Source: CAD feature listing. Evaluate the final solid. Frame: model axes, mm. A direction names the side the tool comes from. Round coordinates to 2 decimals unless told otherwise and drop trailing zeros. Loops run counter-clockwise (first coordinate to the right, second up) from the corner with the lowest first, then second, coordinate; pieces in that order, holes last. Notation, with made-up numbers: M 76,84.5 L 134,84.5 A25 ccw 134,122.5 Z; hole C 5.5,46.25 d6. An arc over 180 degrees is marked long. Answer as a JSON object with one key per item and string values.
from build123d import *

# Parameters (mm, degrees)
PLUS_PLATE_10_X_8_5_X_0_5_SKETCH_W = 10
PLUS_PLATE_10_X_8_5_X_0_5_SKETCH_H = 0.5
PLUS_PLATE_10_X_8_5_X_0_5_DEPTH    = 8.5
SOLDER_TAB_1_5_X_2_5_SKETCH_W      = 1.5
SOLDER_TAB_1_5_X_2_5_SKETCH_H      = 0.5
SOLDER_TAB_1_5_X_2_5_DEPTH         = 2.5


with BuildPart() as part:
    # Plus Plate 10 x 8.5 x 0.5 Sketch → Plus Plate 10 x 8.5 x 0.5 (new body)
    with BuildSketch(Plane(origin=(0, 1.95, 0), x_dir=(1, 0, 0), z_dir=(0, 1, 0))):
        with Locations((14.3, 65.1)):
            Rectangle(PLUS_PLATE_10_X_8_5_X_0_5_SKETCH_W, PLUS_PLATE_10_X_8_5_X_0_5_SKETCH_H)
    extrude(amount=PLUS_PLATE_10_X_8_5_X_0_5_DEPTH)

    # Solder Tab 1.5 x 2.5 Sketch → Solder Tab 1.5 x 2.5 (add)
    with BuildSketch(Plane(origin=(0, 10.45, 0), x_dir=(1, 0, 0), z_dir=(0, 1, 0))):
        with Locations((14.3, 65.1)):
            Rectangle(SOLDER_TAB_1_5_X_2_5_SKETCH_W, SOLDER_TAB_1_5_X_2_5_SKETCH_H)
    extrude(amount=SOLDER_TAB_1_5_X_2_5_DEPTH)

    # Dimple 0.9 Sketch → Dimple 0.9 (revolve)
    with BuildSketch(Plane(origin=(0, 6.95, 0), x_dir=(1, 0, 0), z_dir=(0, 1, 0))):
        with BuildLine():
            Line((14.3, 64.85), (16.8, 64.85))
            ThreePointArc((16.8, 64.85), (15.628533026, 64.181852707), (14.3, 63.95))
            Line((14.3, 63.95), (14.3, 64.85))
        make_face()
    revolve(axis=Axis((14.3, 6.95, -65.85), (0, 0, 1)))


solid = part.part
Item 1: Access query for faces 1 (the flat face through (14, 6, -65.35)), 2 (the flat face through (14, 4, -64.85)). Directions: +Z, -Z, +X, -X, +Y, -Y. A direction counts if a zero-diameter tool reaches every point of the face in a straight line with its end or side. Return the directions, or none.
Answer sheet:
{"face 1": "-Z, +X, -X, +Y, -Y", "face 2": "+Z"}
Item 2: Section C-C on x = 15.5. Return the cut outline in (y, z).
Answer sheet:
{"outline": "M 1.95,-65.35 L 10.45,-65.35 L 10.45,-64.85 L 9.14,-64.85 A3.73 ccw 4.76,-64.85 L 1.95,-64.85 Z"}
Item 3: Line query: probe 1 along Y at (x, z) = (19, -64.9); probe 2 along Z at (x, y) = (13.25, 2.5); probe 3 along X at (y, z) = (10.5, -65.15). Output: solid intervals per line, ascending. Write a range as from..to.
Answer sheet:
{"probe 1": "y = 1.95..10.45", "probe 2": "z = -65.35..-64.85", "probe 3": "x = 13.55..15.05"}
Item 4: Section B-B on y = 5.75. Return the cut outline in (x, z), then the cut area to 3 significant figures.
Answer sheet:
{"outline": "M 9.3,-65.35 L 19.3,-65.35 L 19.3,-64.85 L 16.49,-64.85 A3.73 ccw 12.11,-64.85 L 9.3,-64.85 Z", "area": "7.13 mm²"}
Item 5: Section D-D on x = 10.5. Return the cut outline in (y, z), then the cut area to 3 significant figures.
Answer sheet:
{"outline": "M 1.95,-65.35 L 10.45,-65.35 L 10.45,-64.85 L 1.95,-64.85 Z", "area": "4.25 mm²"}
Item 6: Contact query for flat-ended pins moving along their axis: pin 1 Ø0.6 at (y, z) = (11.5, -65) entering from -X; pin 2 Ø3 at (x, y) = (11.5, 5) entering from +Z. Output: stop coordinate, or through.
Answer sheet:
{"pin 1": "stops at x = 13.55", "pin 2": "stops at z = -64.45"}
Item 7: Section A-A on z = -65.05. Return the cut outline in (x, y), then the cut area to 4 significant figures.
Answer sheet:
{"outline": "M 9.3,1.95 L 19.3,1.95 L 19.3,10.45 L 15.05,10.45 L 15.05,12.95 L 13.55,12.95 L 13.55,10.45 L 9.3,10.45 Z", "area": "88.75 mm²"}
